Build history of the part. All positions in model axes, mm. A direction names the side the tool comes from. Round coordinates to 2 decimals unless told otherwise and drop trailing zeros. Order: outer loops, then holes, each group sorted by start corner. A loop starts at its lowest first (then second) coordinate and runs counter-clockwise, first axis right, second up. Notation, with made-up numbers: (-33.5, -5) - (9.5, -5) arc R23 cw to (9.5, 19) - close; hole circle Ø5 at (73.25, -28.5). An arc over 180 degrees is marked (long way). One line per question, with ' | ' between items. Start each with the question number.
from build123d import *

# Parameters (mm, degrees)
SKETCH1_W                           = 15
SKETCH1_H                           = 18
BOSS_EXTRUDE1_DEPTH                 = 10
SKETCH2_R                           = 2.5
CUT_EXTRUDE1_DEPTH                  = 11
SKETCH3_R                           = 3.05
CUT_EXTRUDE2_DEPTH                  = 16
TALADRO_ROSCADO_M31_D               = 2.5
TALADRO_ROSCADO_M31_DEPTH           = 4
TALADRO_ROSCADO_M31_TIP             = 0.751075774
DI_METRO_DE_TALADRO_2_8_2_8_1_D     = 2
DI_METRO_DE_TALADRO_2_8_2_8_1_DEPTH = 12
DI_METRO_DE_TALADRO_2_8_2_8_1_TIP   = 0.600860619


with BuildPart() as part:
    # Sketch1 → Boss-Extrude1 (new body)
    with BuildSketch(Plane.XY):
        Rectangle(SKETCH1_W, SKETCH1_H)
    extrude(amount=BOSS_EXTRUDE1_DEPTH)

    # Sketch2 → Cut-Extrude1 (cut, through all)
    with BuildSketch(Plane(origin=(0, 0, 0), x_dir=(-1, 0, 0), z_dir=(0, 0, -1))):
        with Locations((0, -2)):
            Circle(SKETCH2_R)
    extrude(amount=-CUT_EXTRUDE1_DEPTH, mode=Mode.SUBTRACT)

    # Sketch3 → Cut-Extrude2 (cut, through all)
    with BuildSketch(Plane(origin=(7.5, 0, 0), x_dir=(0, 0, -1), z_dir=(1, 0, 0))):
        with Locations((-4, 4.75)):
            Circle(SKETCH3_R)
    extrude(amount=-CUT_EXTRUDE2_DEPTH, mode=Mode.SUBTRACT)

    # Taladro roscado M31
    with Locations(Plane(origin=(-2.648652683, -2.97524228, 10), x_dir=(1, 0, 0), z_dir=(0, 0, 1))):
        with Locations((7.148652683, 7.72524228), (7.148652683, -3.82475772)):
            Hole(TALADRO_ROSCADO_M31_D / 2, depth=TALADRO_ROSCADO_M31_DEPTH)
            with Locations((0, 0, -(TALADRO_ROSCADO_M31_DEPTH + TALADRO_ROSCADO_M31_TIP / 2))):  # 118° drill point
                Cone(0, TALADRO_ROSCADO_M31_D / 2, TALADRO_ROSCADO_M31_TIP, mode=Mode.SUBTRACT)

    # Diámetro de taladro Ø2.8 (2.8)1
    with Locations(Plane(origin=(7.5, -6.8, 6.5), x_dir=(0, 0, 1), z_dir=(1, 0, 0))):
        with Locations((0, 0)):
            Hole(DI_METRO_DE_TALADRO_2_8_2_8_1_D / 2, depth=DI_METRO_DE_TALADRO_2_8_2_8_1_DEPTH)
            with Locations((0, 0, -(DI_METRO_DE_TALADRO_2_8_2_8_1_DEPTH + DI_METRO_DE_TALADRO_2_8_2_8_1_TIP / 2))):  # 118° drill point
                Cone(0, DI_METRO_DE_TALADRO_2_8_2_8_1_D / 2, DI_METRO_DE_TALADRO_2_8_2_8_1_TIP, mode=Mode.SUBTRACT)


solid = part.part
Item 1: Slice it at A-A (y = -2). Write the cut outline in (x, z), plus the area to 3 significant figures.
Item 2: Pull direction Z, two halves, no side cores. Call faces 4 (the face through (4.7, -6.88, 5.38)), 5 (the face through (6.466, -7.1, 5.546)), 6 (the face through (-7.5, 0, 5)): released by +Z, released by -Z, zero draft, split by the parting line, or undercut.
Item 3: Slice it at D-D (x = 1.75). Write the cut outline in (y, z), plus the area to 3 significant figures.
Item 4: 3-axis set-ups, long thin cutter, end or side, ignore diameter. For faces 1 (the face through (3.31, -6.42, 8.42)), 2 (the face through (-0.254, -7.1, 5.546)), 3 (the face through (-1.15, -4.22, 4.93)): which of +Z, -Z, +X, -X, +Y, -Y reach the whole face in a straight line?
Item 5: Pin check, flat tips, straight feed: pin 1 (5 mm diameter, centred on x = -2.5, y = -4.5, fed in from -Z); pin 2 (2 mm diameter, centred on x = -0.5, y = -3, fed in from -Z). Stop position of each tip, or through.
Item 6: Slice it at C-C (x = 6.25). Write the cut outline in (y, z), plus the area to 3 significant figures.
Item 7: Slice it at B-B (z = 2.75). Write the cut outline in (x, y), plus the area to 3 significant figures.
Item 8: Wall check: line 1 along Y through (x, z) = (4.5, 8.4); line 2 along X through (y, z) = (-6.8, 8.8); line 3 along Z through (x, y) = (-1.5, -6.8). Give the ranges that are in metal, low to high. Write a range as [from, to].
A:
1) outline: (-7.5, 0) - (-2.5, 0) - (-2.5, 10) - (-7.5, 10) - close; (2.5, 0) - (7.5, 0) - (7.5, 10) - (2.5, 10) - close | area: 100 mm^2
2) face 4: released by +Z | face 5: undercut | face 6: zero draft
3) outline: (-9, 0) - (-3.79, 0) - (-3.79, 10) - (-9, 10) - close; (-0.21, 0) - (9, 0) - (9, 10) - (-0.21, 10) - close; hole circle Ø2 at (-6.8, 6.5); hole circle Ø6.1 at (4.75, 4) | area: 112 mm^2
4) face 1: +Z | face 2: +X | face 3: +Z, -Z
5) pin 1: z = 0 | pin 2: through
6) outline: (-9, 0) - (9, 0) - (9, 10) - (-9, 10) - close; hole circle Ø2 at (-6.8, 6.5); hole circle Ø6.1 at (4.75, 4) | area: 148 mm^2
7) outline: (-7.5, -9) - (7.5, -9) - (7.5, 1.97) - (-7.5, 1.97) - close; (-7.5, 7.53) - (7.5, 7.53) - (7.5, 9) - (-7.5, 9) - close; hole circle Ø5 at (0, -2) | area: 167 mm^2
8) line 1: [-9, -8.05], [-5.55, 3.5], [6, 9] | line 2: [-7.5, 3.25], [5.75, 7.5] | line 3: [0, 5.5], [7.5, 10]
